Can you work these out from the model? Positions are in its coordinate system, mm. Face numbers are marked on the shaded views. Round coordinates to 2 decimals unless told otherwise and drop trailing zeros. Loops run counter-clockwise (first coordinate to the right, second up) from the corner with the lowest first, then second, coordinate; pieces in that order, holes last.
from build123d import *

# Parameters (mm, degrees)
SKETCH1_R                    = 21
BOSS_EXTRUDE1_DEPTH          = 10
SKETCH2_R                    = 12.5
BOSS_EXTRUDE2_DEPTH          = 15
SKETCH3_R                    = 5
CUT_EXTRUDE1_DEPTH           = 39.820097888
SKETCH4_R                    = 2.5
CUT_EXTRUDE2_DEPTH           = 39.820097888
FILLET1_R                    = 0.5
CHAMFER2_SIZE                = 0.75
CIRPATTERN2_COUNT            = 6
CHAMFER2_OF_CIRPATTERN2_SIZE = 0.75


with BuildPart() as part:
    # Sketch1 → Boss-Extrude1 (new body)
    with BuildSketch(Plane.XY):
        Circle(SKETCH1_R)
    extrude(amount=BOSS_EXTRUDE1_DEPTH)

    # Sketch2 → Boss-Extrude2 (add)
    with BuildSketch(Plane.XY.offset(10)):
        Circle(SKETCH2_R)
    extrude(amount=BOSS_EXTRUDE2_DEPTH)

    # Sketch3 → Cut-Extrude1 (cut, through all)
    with BuildSketch(Plane.XY.offset(25)):
        Circle(SKETCH3_R)
    extrude(amount=-CUT_EXTRUDE1_DEPTH, mode=Mode.SUBTRACT)

    # Sketch4 → Cut-Extrude2 (cut, through all)
    with BuildSketch(Plane(origin=(0, 0, 0), x_dir=(-1, 0, 0), z_dir=(0, 0, -1))):
        with Locations((0, 17)):
            Circle(SKETCH4_R)
    cut_extrude2 = extrude(amount=-CUT_EXTRUDE2_DEPTH, mode=Mode.SUBTRACT)

    # Fillet1
    fillet1_edges = [part.edges().sort_by_distance(p)[0] for p in [
        (-21, 0, 10),
        (-12.5, 0, 10),
        (-12.5, 0, 25),
    ]]
    fillet(fillet1_edges, radius=FILLET1_R)

    # Chamfer2
    chamfer2_edges = [part.edges().sort_by_distance(p)[0] for p in [
        (2.5, 17, 10),
    ]]
    chamfer(chamfer2_edges, length=CHAMFER2_SIZE)

    # CirPattern2: Cut-Extrude2 ×6 about axis
    cirpattern2_axis = Axis((0, 0, 0), (0, 0, 1))
    for i in range(1, CIRPATTERN2_COUNT):
        add(cut_extrude2.rotate(cirpattern2_axis, i * 360 / CIRPATTERN2_COUNT), mode=Mode.SUBTRACT)

    # Chamfer2 of CirPattern2
    chamfer2_of_cirpattern2_edges = [part.edges().sort_by_distance(p)[0] for p in [
        (-13.472431864, 10.665063509, 10),
        (-15.972431864, -6.334936491, 10),
        (-2.5, -17, 10),
        (13.472431864, -10.665063509, 10),
        (15.972431864, 6.334936491, 10),
    ]]
    chamfer(chamfer2_of_cirpattern2_edges, length=CHAMFER2_OF_CIRPATTERN2_SIZE)


solid = part.part
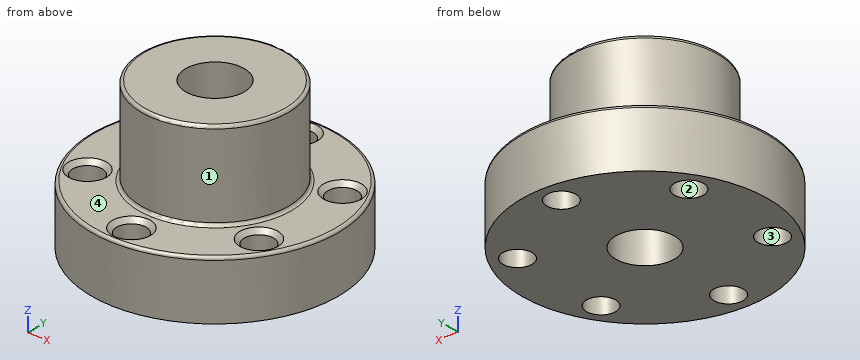
(1) If we section it at C-C, the plane z = 3.75: List the corners of the cut face in (x, y) for me, then the cut area to 3 significant figures.
Worked answers:
outline: circle Ø42 at (0, 0); hole circle Ø5 at (-14.72, -8.5); hole circle Ø5 at (-14.72, 8.5); hole circle Ø10 at (0, 0); hole circle Ø5 at (0, -17); hole circle Ø5 at (0, 17); hole circle Ø5 at (14.72, -8.5); hole circle Ø5 at (14.72, 8.5)
area: 1,190 mm2
(2) Will these pins go through, and if not, where does the flat tip stop? P1, Ø12, axis at x = -8.5, z = 8, coming from the -Y side; P2, Ø6, axis at x = 0, y = 0, coming from the +Z side; P3, Ø4, axis at y = 13, z = 18, coming from the +X side; P4, Ø10, axis at y = -9.5, z = 14, coming from the -X side.
Worked answers:
P1: stops at y = -20.85
P2: passes through
P3: stops at x = 5.94
P4: stops at x = -19.78
(3) If we section it at A-A, the plane x = 0: State how many separate pieces and enclosed holes the cut face has, then the cut area to 3 significant figures.
Worked answers:
separate pieces: 4
enclosed holes: 0
area: 444 mm2
(4) If we mould it in two halves opening along X, with no side actions, what happens to the marked faces 1, 2, 3 and 4? For each: released by +X, released by -X, zero draft, split by the parting line, or undercut.
Worked answers:
face 1: split by the parting line
face 2: undercut
face 3: undercut
face 4: zero draft
(5) If we section it at B-B, the plane y = 0: List the corners of the cut face in (x, z) for me.
Worked answers:
outline: (-21, 0) - (-5, 0) - (-5, 25) - (-12, 25) arc R0.5 ccw to (-12.5, 24.5) - (-12.5, 10.5) arc R0.5 cw to (-13, 10) - (-20.5, 10) arc R0.5 ccw to (-21, 9.5) - close; (5, 0) - (21, 0) - (21, 9.5) arc R0.5 ccw to (20.5, 10) - (13, 10) arc R0.5 cw to (12.5, 10.5) - (12.5, 24.5) arc R0.5 ccw to (12, 25) - (5, 25) - close
(6) If we section it at D-D, the plane z = 18.25: List the corners of the cut face in (x, y) for me, then the cut area to 3 significant figures.
Worked answers:
outline: circle Ø25 at (0, 0); hole circle Ø10 at (0, 0)
area: 412 mm2
(7) If I drill on line 1 (Y direction, x = 0, z = 6.25); line 2 (Y direction, x = -1.5, z = 1.5); line 3 (Y direction, x = 14, z = 2.5), over which ranges is the centre line in solid material (lowest first)?
Worked answers:
line 1: y = -21 to -19.5, -14.5 to -5, 5 to 14.5, 19.5 to 21
line 2: y = -20.95 to -19, -15 to -4.77, 4.77 to 15, 19 to 20.95
line 3: y = -15.65 to -10.89, -6.11 to 6.11, 10.89 to 15.65
